from build123d import *

# Parameters (mm, degrees)
F0_W     = 127.461821
F0_H     = 58.419999
F1_DEPTH = 25.4
F2_T     = -2.54
F4_D     = 4
F5_W     = 22.663121
F5_H     = 17.466478
F6_DEPTH = 21.844
F7_W     = 47.276701
F7_H     = 17.408888
F7_W_2   = 45.647759
F7_W_3   = 22.663121
F8_DEPTH = 3.048


with BuildPart() as f1:
    # F0 (on Front) → F1 (new body)
    with BuildSketch(Plane.XZ):
        with Locations((1.847274, 26.785453)):
            Rectangle(F0_W, F0_H)
    extrude(amount=F1_DEPTH)

    # F2
    f2_openings = [f1.faces().sort_by_distance(p)[0] for p in [
        (1.847275, -25.4, 26.785454),
    ]]
    offset(amount=F2_T, openings=f2_openings)

    # F4 (through all)
    with Locations(Plane(origin=(0, 0, 0), x_dir=(-1, 0, 0), z_dir=(0, 1, 0))):
        with Locations((51.723637, 5.195455)):
            Hole(F4_D / 2)

    # F5 (on face) → F6 (join)
    with BuildSketch(Plane(origin=(0, 0, -2.424546), x_dir=(1, 0, 0), z_dir=(0, 0, -1))):
        with Locations((1.726462, 12.215246)):
            Rectangle(F5_W, F5_H)
    extrude(amount=F6_DEPTH)

    # F7 (on face) → F8 (join)
    with BuildSketch(Plane(origin=(0, 0, -24.268546), x_dir=(1, 0, 0), z_dir=(0, 0, -1))):
        with Locations((36.696372, 12.244041)):
            Rectangle(F7_W, F7_H)
        with Locations((-32.428978, 12.244041)):
            Rectangle(F7_W_2, F7_H)
        with Locations((1.726462, 12.244041)):
            Rectangle(F7_W_3, F7_H)
    extrude(amount=F8_DEPTH)


solid = f1.part
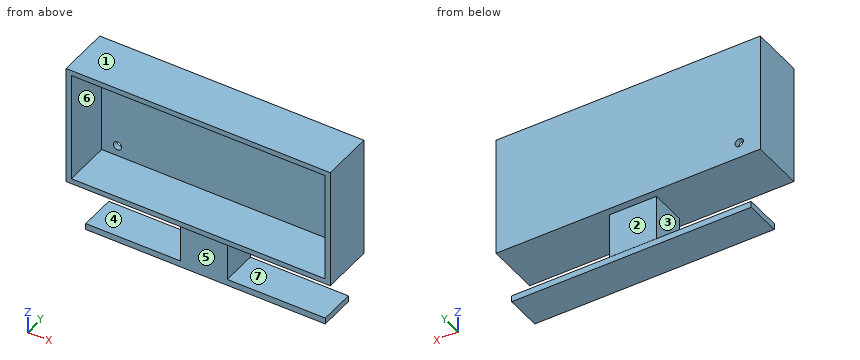
Could you check a few things on this model? Use its own coordinates, in mm. Face numbers are marked on the shaded views. A direction names the side the tool comes from. Give positions to 0.01 mm unless a question says otherwise; leave off trailing zeros. Write each loop counter-clockwise with the first axis right and the second up, starting at its lowest first coordinate (ties: lowest second). Pieces come first, ordered by that corner, then holes. Notation, with made-up numbers: (-31.75, -1) - (22.25, -1) arc R25 ccw to (22.25, 19) - close; hole circle Ø3 at (26.25, 76). An arc over 180 degrees is marked (long way). Use CSV: the item, a comma, the result in double quotes. Start each with the question number.
Item 1: If we mould it in two halves opening along Z, with no side actions, what happens to the marked faces 1, 2 and 3? For each: pulls with the +Z half, pulls with the -Z half, needs draft (parallel to the pull), parting line crosses it, or undercut.
Item 2: I want a section at A-A, the plane x = 17. Please give me the cut outline in (y, z), then the cut area to 3 significant figures.
Item 3: I want a section at C-C, the plane z = 24. Please give me the cut outline in (x, y).
Item 4: I want a section at D-D, the plane x = 3. Please give me the cut outline in (y, z), then the cut area to 3 significant figures.
Item 5: I'm going to push flat-ended pins straight in: pin 1 (5 mm diameter, centred on y = -10, z = -7, fed in from -X); pin 2 (16 mm diameter, centred on x = 13, z = 27.5, fed in from -Y); pin 3 (11 mm diameter, centred on x = 1, z = -18, fed in from +Y); pin 4 (1 mm diameter, centred on x = 17.5, z = 25, fed in from +Y). Where does each tip first touch, or does it pass through?
Item 6: For the marked faces 4, 5, 6 and 7, which set-ups out of +Z, -Z, +X, -X, +Y, -Y let a thin tool reach every point of the face, with its end or its side?
Item 7: If I drill on line 1 along Z through (x, y) = (-22.5, -17.75); line 2 along Z through (x, y) = (-2.5, -18); line 3 along X through (y, z) = (-17.25, 18), over which ranges is the centre line in solid material (lowest first)?
Item 8: I want a section at B-B, the plane y = -18.75. Please give me the cut outline in (x, z).
Findings:
1,face 1,"pulls with the +Z half"
1,face 2,"needs draft"
1,face 3,"undercut"
2,outline,"(-25.4, -2.42) - (0, -2.42) - (0, 56) - (-25.4, 56) - (-25.4, 53.46) - (-2.54, 53.46) - (-2.54, 0.12) - (-25.4, 0.12) - close; (-20.95, -27.32) - (-3.54, -27.32) - (-3.54, -24.27) - (-20.95, -24.27) - close"
2,area,"318 mm2"
3,outline,"(-61.88, -25.4) - (-59.34, -25.4) - (-59.34, -2.54) - (63.04, -2.54) - (63.04, -25.4) - (65.58, -25.4) - (65.58, 0) - (-61.88, 0) - close"
4,outline,"(-25.4, -2.42) - (-20.95, -2.42) - (-20.95, -27.32) - (-3.54, -27.32) - (-3.54, -24.27) - (-3.48, -24.27) - (-3.48, -2.42) - (0, -2.42) - (0, 56) - (-25.4, 56) - (-25.4, 53.46) - (-2.54, 53.46) - (-2.54, 0.12) - (-25.4, 0.12) - close"
4,area,"699 mm2"
5,pin 1,"stops at x = -9.61"
5,pin 2,"stops at y = -2.54"
5,pin 3,"stops at y = -3.48"
5,pin 4,"stops at y = 0"
6,face 4,"-X, +Y, -Y"
6,face 5,"-Z, +X, -X, -Y"
6,face 6,"-Y"
6,face 7,"+X, +Y, -Y"
7,line 1,"z = -27.32 to -24.27, -2.42 to 0.12, 53.46 to 56"
7,line 2,"z = -27.32 to 0.12, 53.46 to 56"
7,line 3,"x = -61.88 to -59.34, 63.04 to 65.58"
8,outline,"(-61.88, -2.42) - (-9.61, -2.42) - (-9.61, -24.27) - (-55.25, -24.27) - (-55.25, -27.32) - (60.33, -27.32) - (60.33, -24.27) - (13.06, -24.27) - (13.06, -2.42) - (65.58, -2.42) - (65.58, 56) - (-61.88, 56) - close; hole (-59.34, 0.12) - (63.04, 0.12) - (63.04, 53.46) - (-59.34, 53.46) - close"
